Here's how the part is built. I have some questions about the finished solid (model axes, mm). A direction names the side the tool comes from. Round coordinates to 2 decimals unless told otherwise and drop trailing zeros. Loops run counter-clockwise (first coordinate to the right, second up) from the corner with the lowest first, then second, coordinate; pieces in that order, holes last. Notation, with made-up numbers: M -36,19 L 11,19 A23 cw 11,39 Z; hole C 15,63 d7. An arc over 180 degrees is marked long. Answer as a JSON object with one key per item and string values.
from build123d import *

# Parameters (mm, degrees)
SKETCH1_R                     = 9
BOSS_EXTRUDE1_DEPTH           = 20
BOSS_EXTRUDE1_TAPER           = 9
BOSS_EXTRUDE1_OTHER_WAY_DEPTH = 30
SKETCH1_4_R                   = 7
SKETCH2_R                     = 4
SKETCH1_5_R                   = 7
CUT_EXTRUDE1_DEPTH            = 5
BOSS_EXTRUDE3_DEPTH           = 3


with BuildPart() as part:
    # Sketch1 → Boss-Extrude1 (new body)
    with BuildSketch(Plane(origin=(0, 0, 0), x_dir=(1, 0, 0), z_dir=(0, 1, 0))):
        with Locations(Location((0, 0, 0), (0, 0, 270))):
            Circle(SKETCH1_R)
    extrude(amount=-BOSS_EXTRUDE1_DEPTH, taper=BOSS_EXTRUDE1_TAPER)

    # Sketch1 → Boss-Extrude1 other way (add)
    with BuildSketch(Plane(origin=(0, 0, 0), x_dir=(1, 0, 0), z_dir=(0, 1, 0))):
        with Locations(Location((0, 0, 0), (0, 0, 270))):
            Circle(SKETCH1_R)
    extrude(amount=BOSS_EXTRUDE1_OTHER_WAY_DEPTH)

    # SurfaceCut1
    split(bisect_by=Plane(origin=(0, 0, 0), x_dir=(0, 0, -1), z_dir=(0.5735764363510473, 0.819152044288991, -1.9675099965776456e-15)), keep=Keep.BOTTOM)

    # Sketch1<4> → Cut-Loft1 section 0
    with BuildSketch(Plane(origin=(0, 0, 0), x_dir=(1, 0, 0), z_dir=(0, 1, 0))):
        Circle(SKETCH1_4_R)
    # Sketch2 → Cut-Loft1 section 1
    with BuildSketch(Plane.XZ.offset(20)):
        Circle(SKETCH2_R)
    loft(mode=Mode.SUBTRACT)

    # Sketch1<5> → Cut-Extrude1 (cut)
    with BuildSketch(Plane(origin=(0, 0, 0), x_dir=(1, 0, 0), z_dir=(0, 1, 0))):
        Circle(SKETCH1_5_R)
    extrude(amount=CUT_EXTRUDE1_DEPTH, mode=Mode.SUBTRACT)

    # Sketch3 → Boss-Extrude3 (add)
    with BuildSketch(Plane.XZ.offset(20)):
        with BuildLine():
            ThreePointArc((0, -5.832311194), (-5.832311194, 0), (0, 5.832311194))
            Line((0, 5.832311194), (-17, 5.832311194))
            Line((-17, 5.832311194), (-17, -5.832311194))
            Line((-17, -5.832311194), (0, -5.832311194))
        make_face()
    extrude(amount=-BOSS_EXTRUDE3_DEPTH)


solid = part.part
Item 1: If we mould it in two halves opening along Y, with no side actions, what happens to faces 1 (the face through (-11, -17, 0)), 2 (the face through (-8, -19, 5.832)), 3 (the face through (-8, -20, 0)), 4 (the face through (-5.14, -12.36, -0.23))? For each: pulls with the +Y half, pulls with the -Y half, needs draft (parallel to the pull), parting line crosses it, or undercut.
Resolved:
{"face 1": "undercut", "face 2": "needs draft", "face 3": "pulls with the -Y half", "face 4": "pulls with the +Y half"}
Item 2: On a 3-axis mill with a long thin cutter (end or side, diameter ignored), from which of +Z, -Z, +X, -X, +Y, -Y can I reach the whole of each face in a straight line? I mean faces 5 (the face through (-9, -19, -5.832)), 6 (the face through (-9, 2, 0)), 7 (the face through (-7, 2, 0)), 8 (the face through (-6.875, -12.362, -1.527)). Say none if no direction works.
Resolved:
{"face 5": "-Z, -X, -Y", "face 6": "-X, +Y", "face 7": "+X, +Y", "face 8": "none"}
Item 3: I want a section at C-C, the plane y = -11. Please give me the cut outline in (x, z), then the cut area to 3 significant figures.
Resolved:
{"outline": "C 0,0 d14.52; hole C 0,0 d10.7", "area": "75.6 mm²"}
Item 4: Please list where these lines run through material, in increasing order: probe 1 along Z at (x, y) = (-4.5, -17.5); probe 2 along Z at (x, y) = (-3.75, -4); probe 3 along Z at (x, y) = (-4.5, -8.5). Write a range as from..to.
Resolved:
{"probe 1": "-5.83..5.83", "probe 2": "-7.48..-5.19, 5.19..7.48", "probe 3": "-6.19..-3.54, 3.54..6.19"}
Item 5: I want a section at A-A, the plane y = -14. Please give me the cut outline in (x, z).
Resolved:
{"outline": "C 0,0 d13.57; hole C 0,0 d9.8"}
Item 6: I'm going to push flat-ended pins straight in: pin 1 Ø10 at (x, y) = (-11, 0) entering from +Z; pin 2 Ø5 at (x, y) = (-0.5, -7) entering from -Z; pin 3 Ø0.9 at (x, y) = (-9.5, -18.5) entering from +Z. Where does each tip first touch, or does it pass through?
Resolved:
{"pin 1": "z = 6.71", "pin 2": "z = -8.28", "pin 3": "z = 5.83"}
Item 7: I want a section at B-B, the plane y = 2.5. Please give me the cut outline in (x, z).
Resolved:
{"outline": "M -3.57,-8.26 L -3.57,-6.02 A7 cw -3.57,6.02 L -3.57,8.26 A9 ccw Z"}
